Can you work these out from the model? Positions are in its coordinate system, mm. A direction names the side the tool comes from. Round coordinates to 2 decimals unless told otherwise and drop trailing zeros. Write each loop counter-clockwise with the first axis right and the second up, starting at its lowest first coordinate (ties: lowest second). Pieces come first, ordered by that corner, then holes.
Q1. We'd pull the mould along Y, two halves only. Please class faces 4 (the flat face through (-6, 5, 3)), 5 (the flat face through (-12, 7, 5)), 6 (the flat face through (0, 0, 20)): +Y half, -Y half, draft (parallel to the pull), parting line (faces both ways), or undercut.
Q2. If we section it at D-D (y = -10): Please give me the cut outline in (x, z), plus the area to 3 significant figures.
Q3. Please list where these lines run through material, in increasing order: line 1 along Y through (x, z) = (12, 2.6); line 2 along X through (y, z) = (12.75, 3.25); line 3 along Y through (x, z) = (10, 18.5).
Q4. If we section it at A-A (z = 9): Please give me the cut outline in (x, y), plus the area to 3 significant figures.
Q5. I'm going to push a flat-ended pin straight in: pin 1 Ø1.5 at (x, z) = (6, 3) entering from +Y. Where does the tip first touch, or does it pass through?
Q6. For faces 1 (the cylindrical face through (4.5, 10.1, 4.3)), 2 (the flat face through (12, 7, 5)), 3 (the cylindrical face through (16.026, -11.464, 15.325)), which set-ups out of +Z, -Z, +X, -X, +Y, -Y let a thin tool reach every point of the face, with its end or its side?
Q7. If we section it at B-B (x = 12): Please give me the cut outline in (y, z), plus the area to 3 significant figures.
Q8. If we section it at C-C (y = 2): Please give me the cut outline in (x, z), plus the area to 3 significant figures.
Autodesk Inventor part; units mm, degrees
ref_plane "YZ Plane" through (0, 0, 0) normal (1, 0, 0) x (0, 1, 0)
ref_plane "XZ Plane" through (0, 0, 0) normal (0, 1, 0) x (-1, 0, 0)
ref_plane "XY Plane" through (0, 0, 0) normal (0, 0, 1) x (1, 0, 0)
sketch "Sketch1" plane through (0, 0, 0) normal (0, 0, 1) x (1, 0, 0)
  circle A0 centre (-12, 9) radius 1.5
  line L0 (12, -9) -> (-12, -9) construction
  line L1 (-12, -9) -> (-12, 9) construction
  line L2 (-12, 9) -> (12, 9) construction
  line L3 (12, 9) -> (12, -9) construction
  line L4 (12, -9) -> (-12, 9) construction
  line L5 (-12, -9) -> (12, 9) construction
  circle A1 centre (12, 9) radius 1.5
  circle A2 centre (12, -9) radius 1.5
  circle A3 centre (-12, -9) radius 1.5
  line L6 (17, -15) -> (-17, -15)
  line L7 (-17, -15) -> (-17, 15)
  line L8 (-17, 15) -> (17, 15)
  line L9 (17, 15) -> (17, -15)
  line L10 (17, -15) -> (-17, 15) construction
  line L11 (-17, -15) -> (17, 15) construction
  circle A4 centre (0, 0) radius 4
  circle A5 centre (12, 9) radius 3.5
  circle A6 centre (-12, 9) radius 3.5
  circle A7 centre (-12, -9) radius 3.5
  circle A8 centre (12, -9) radius 3.5
  circle A9 centre (10, 0) radius 1.5
  circle A10 centre (-10, 0) radius 1.5
  line L12 (10, 0) -> (0, 0) construction
  line L13 (0, 0) -> (-10, 0) construction
  point P0 (0, 0)
  dimension "d0" = 3
  dimension "d1" = 24
  dimension "d2" = 18
  dimension "d3" = 3
  dimension "d4" = 3
  dimension "d5" = 3
  dimension "d6" = 34
  dimension "d7" = 30
  dimension "d8" = 8
  dimension "d15" = 2
  dimension "d16" = 2
  dimension "d17" = 2
  dimension "d18" = 2
  dimension "d59" = 3
  dimension "d60" = 10
  dimension "d61" = 10
  dimension "d62" = 3
extrude "Extrusion1" add sketch "Sketch1" along normal blind 20 contours L6 L7 L8 L9 | A4
extrude "Extrusion3" add sketch "Sketch1" along normal blind 5 from surface at 0 contours A5 | A6 | A7 | A8
sketch "Sketch2" plane through (-17, 15, 0) normal (0, 1, 0) x (1, 0, 0)
  circle A0 centre (17, -9) radius 5.3
  line L0 (17, -9) -> (17, 0) construction
  line L1 (17, -9) -> (22.6569, -14.6569) construction
  line L2 (17, -9) -> (25, -9) construction
  circle A1 centre (22.6569, -14.6569) radius 1.5
  circle A2 centre (22.6569, -3.3431) radius 1.5
  circle A3 centre (11.3431, -3.3431) radius 1.5
  circle A4 centre (11.3431, -14.6569) radius 1.5
  line L3 (17, -9) -> (17, 11) construction
  line L4 (20.5261, 0) -> (13.5408, 0) construction
  dimension "d11" = 10.6
  dimension "d12" = 9
  dimension "d21" = 45
  dimension "d22" = 8
  dimension "d23" = 3
  dimension "d26" = 360
  dimension "d49" = 20
  dimension "d50" = 11
extrude "Extrusion2" cut sketch "Sketch2" against normal through all contours A0
extrude "Extrusion4" cut sketch "Sketch2" against normal blind 10 contours A1 | A2 | A3 | A4
sketch "Sketch3" plane through (0, 0, 0) normal (0, 1, 0) x (-1, 0, 0)
  line L0 (-64.168, -21.8863) -> (-22.168, -21.8863)
  line L1 (-22.168, -21.8863) -> (-22.168, 20.1137)
  line L2 (-22.168, 20.1137) -> (-64.168, 20.1137)
  line L3 (-64.168, 20.1137) -> (-64.168, -21.8863)
  line L4 (-64.168, -21.8863) -> (-22.168, 20.1137) construction
  line L5 (-22.168, -21.8863) -> (-64.168, 20.1137) construction
  circle A0 centre (-27.668, 14.6137) radius 1.5
  circle A1 centre (-27.668, -16.3863) radius 1.5
  circle A2 centre (-58.668, -16.3862) radius 1.5
  circle A3 centre (-58.668, 14.6138) radius 1.5
  circle A4 centre (-43.168, -0.8863) radius 11
  circle A5 centre (-43.168, -0.8863) radius 4
  line L6 (-22.168, -17.8863) -> (-26.168, -21.8863)
  line L7 (-22.168, 16.1137) -> (-26.168, 20.1137)
  line L8 (-60.168, -21.8863) -> (-64.168, -17.8863)
  line L9 (-64.168, 16.1137) -> (-60.168, 20.1137)
  circle A6 centre (-43.168, -0.8863) radius 2.5
  point P0 (0, 0)
  dimension "d30" = 42
  dimension "d31" = 31
  dimension "d32" = 31
  dimension "d33" = 31
  dimension "d34" = 31
  dimension "d35" = 3
  dimension "d36" = 3
  dimension "d37" = 3
  dimension "d38" = 3
  dimension "d39" = 22
  dimension "d40" = 8
  dimension "d41" = 4
  dimension "d42" = 4
  dimension "d43" = 4
  dimension "d44" = 4
  dimension "d45" = 4
  dimension "d46" = 4
  dimension "d47" = 4
  dimension "d48" = 5
sketch "Sketch4" plane through (17, -15, 0) normal (1, 0, 0) x (0, 0, -1)
  circle A0 centre (-15, 25) radius 1.5
  line L0 (-20, 0) -> (-20, 30)
  line L1 (0, 30) -> (-20, 30)
  circle A1 centre (-15, 5) radius 1.5
  line L2 (0, 0) -> (-20, 0)
  point P0 (0, 15)
  dimension "d51" = 3
  dimension "d52" = 5
  dimension "d53" = 5
  dimension "d54" = 3
  dimension "d55" = 5
  dimension "d56" = 5
extrude "Extrusion5" cut sketch "Sketch4" against normal blind 5
equation "\"d3\" = d0"
equation "\"d4\" = d0"
equation "\"d5\" = d0"
equation "\"d16\" = d15"
equation "\"d17\" = d15"
equation "\"d18\" = d15"
equation "\"d61\" = d60"
equation "\"d32\" = d31"
equation "\"d33\" = d31"
equation "\"d34\" = d31"
equation "\"d36\" = d35"
equation "\"d37\" = d35"
equation "\"d38\" = d35"
equation "\"d42\" = d41"
equation "\"d43\" = d41"
equation "\"d44\" = d41"
equation "\"d45\" = d41"
equation "\"d46\" = d41"
equation "\"d47\" = d41"
equation "\"d54\" = d51"
equation "\"d55\" = d52"
equation "\"d56\" = d53"
properties part number "ZX Axis Carriage"
A:
1. face 4: +Y half
1. face 5: undercut
1. face 6: draft
2. outline: (-17, 0) - (-13.12, 0) - (-13.12, 5) - (-15.35, 5) - (-15.35, 20) - (-17, 20) - close; (-10.88, 0) - (10.88, 0) - (10.88, 5) - (8.65, 5) - (8.65, 20) - (-8.65, 20) - (-8.65, 5) - (-10.88, 5) - close; (13.12, 0) - (17, 0) - (17, 13.5) - (15.35, 13.5) - (15.35, 5) - (13.12, 5) - close; (15.35, 16.5) - (17, 16.5) - (17, 20) - (15.35, 20) - close; hole circle Ø10.6 at (0, 9)
2. area: 363 mm2
3. line 1: y = -15 to -10.5, -7.5 to 7.5, 10.5 to 15
3. line 2: x = -17 to -7.15, -4.16 to 4.16, 7.15 to 17
3. line 3: y = -15 to -11.87, -6.13 to -1.5, 1.5 to 6.13, 11.87 to 15
4. outline: (-17, -15) - (-5.3, -15) - (-5.3, 15) - (-17, 15) - close; (5.3, -15) - (17, -15) - (17, 15) - (5.3, 15) - close; hole circle Ø7 at (-12, -9); hole circle Ø7 at (-12, 9); hole circle Ø3 at (-10, 0); hole circle Ø7 at (12, -9); hole circle Ø3 at (10, 0); hole circle Ø7 at (12, 9)
4. area: 534 mm2
5. pin 1: stops at y = 5
6. face 1: +Y
6. face 2: +Z
6. face 3: +X
7. outline: (-15, 0) - (-10.5, 0) - (-10.5, 5) - (-12.5, 5) - (-12.5, 20) - (-15, 20) - close; (-7.5, 0) - (7.5, 0) - (7.5, 5) - (5.5, 5) - (5.5, 20) - (-5.5, 20) - (-5.5, 5) - (-7.5, 5) - close; (10.5, 0) - (15, 0) - (15, 20) - (12.5, 20) - (12.5, 5) - (10.5, 5) - close
7. area: 360 mm2
8. outline: (-17, 0) - (17, 0) - (17, 20) - (-17, 20) - close; hole circle Ø10.6 at (0, 9)
8. area: 592 mm2
